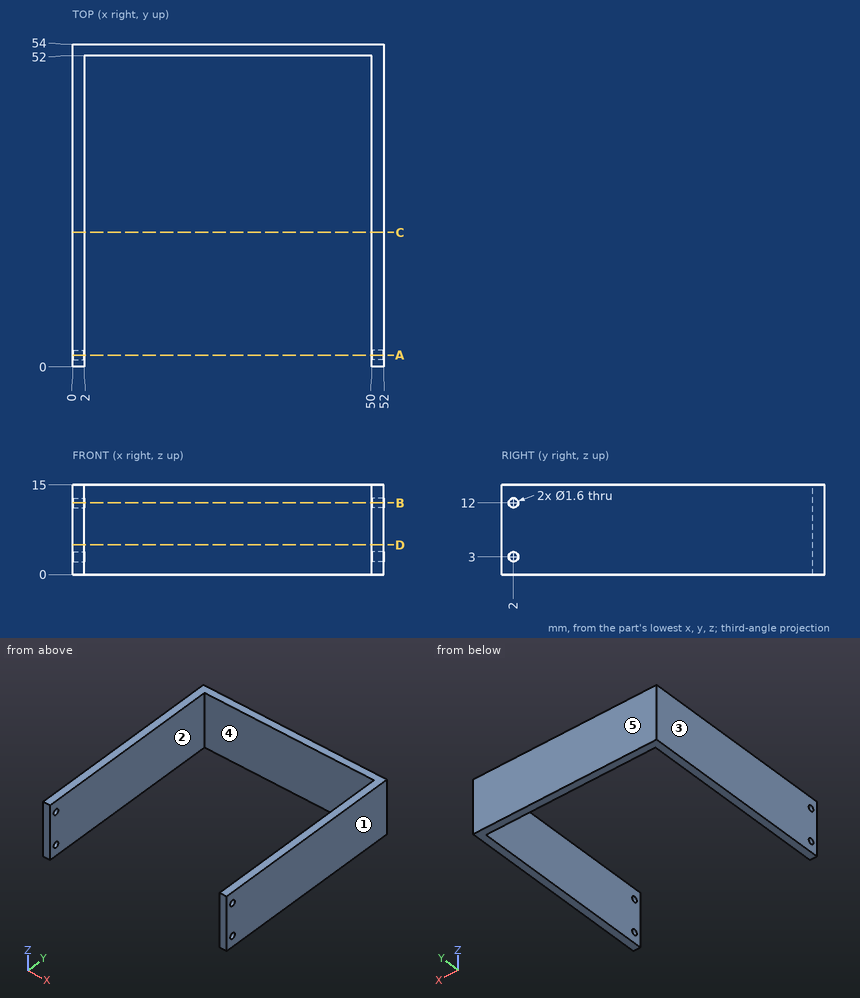
Drawing for the job (mm, zero at the part's lowest x, y, z). A direction names the side the tool comes from. Give positions to 0.01 mm unless a question says otherwise; leave off trailing zeros. Order: outer loops, then holes, each group sorted by start corner. A loop starts at its lowest first (then second) coordinate and runs counter-clockwise, first axis right, second up. Notation, with made-up numbers: M 77,-16 L 111,-16 A25 ccw 111,20 Z; hole C -12.75,-37.75 d2. An arc over 180 degrees is marked long. Put each result on its own line as item: value. Start each with the question number.
(1) Saw through at D-D, the plane z = 5. Write the cut outline in (x, y), then the cut area to 3 significant figures.
(2) Saw through at C-C, the plane y = 22.5. Write the cut outline in (x, z), then the cut area to 3 significant figures.
(3) Drill centre lines: line 1 along X through (y, z) = (12.5, 13); line 2 along Y through (x, z) = (51.65, 12); line 3 along Y through (x, z) = (46, 7). Where is each one in solid material? Low to high.
(4) Which spindle directions (+Z, -Z, +X, -X, +Y, -Y) get a long thin tool onto all of the face, cutting with end or side? Do the marked faces 1 and 2. Say none if no direction does.
(5) Mould opens along X. For the marked faces 3, 4 and 5 say: +X half, -X half, draft (parallel to the pull), parting line (faces both ways), or undercut.
(6) Saw through at A-A, the plane y = 2. Write the cut outline in (x, z), then the cut area to 3 significant figures.
(7) Saw through at B-B, the plane z = 12. Write the cut outline in (x, y).
Check result:
1. outline: M 0,0 L 2,0 L 2,52 L 50,52 L 50,0 L 52,0 L 52,54 L 0,54 Z
1. area: 312 mm2
2. outline: M 0,0 L 2,0 L 2,15 L 0,15 Z; M 50,0 L 52,0 L 52,15 L 50,15 Z
2. area: 60.0 mm2
3. line 1: x = 0 to 2, 50 to 52
3. line 2: y = 0 to 1.2, 2.8 to 54
3. line 3: y = 52 to 54
4. face 1: +Z, -Z, +X, +Y, -Y
4. face 2: +Z, -Z, -Y
5. face 3: -X half
5. face 4: undercut
5. face 5: draft
6. outline: M 0,0 L 2,0 L 2,2.2 L 0,2.2 Z; M 0,3.8 L 2,3.8 L 2,11.2 L 0,11.2 Z; M 0,12.8 L 2,12.8 L 2,15 L 0,15 Z; M 50,0 L 52,0 L 52,2.2 L 50,2.2 Z; M 50,3.8 L 52,3.8 L 52,11.2 L 50,11.2 Z; M 50,12.8 L 52,12.8 L 52,15 L 50,15 Z
6. area: 47.2 mm2
7. outline: M 0,0 L 2,0 L 2,1.2 L 0,1.2 Z; M 0,2.8 L 2,2.8 L 2,52 L 50,52 L 50,2.8 L 52,2.8 L 52,54 L 0,54 Z; M 50,0 L 52,0 L 52,1.2 L 50,1.2 Z
